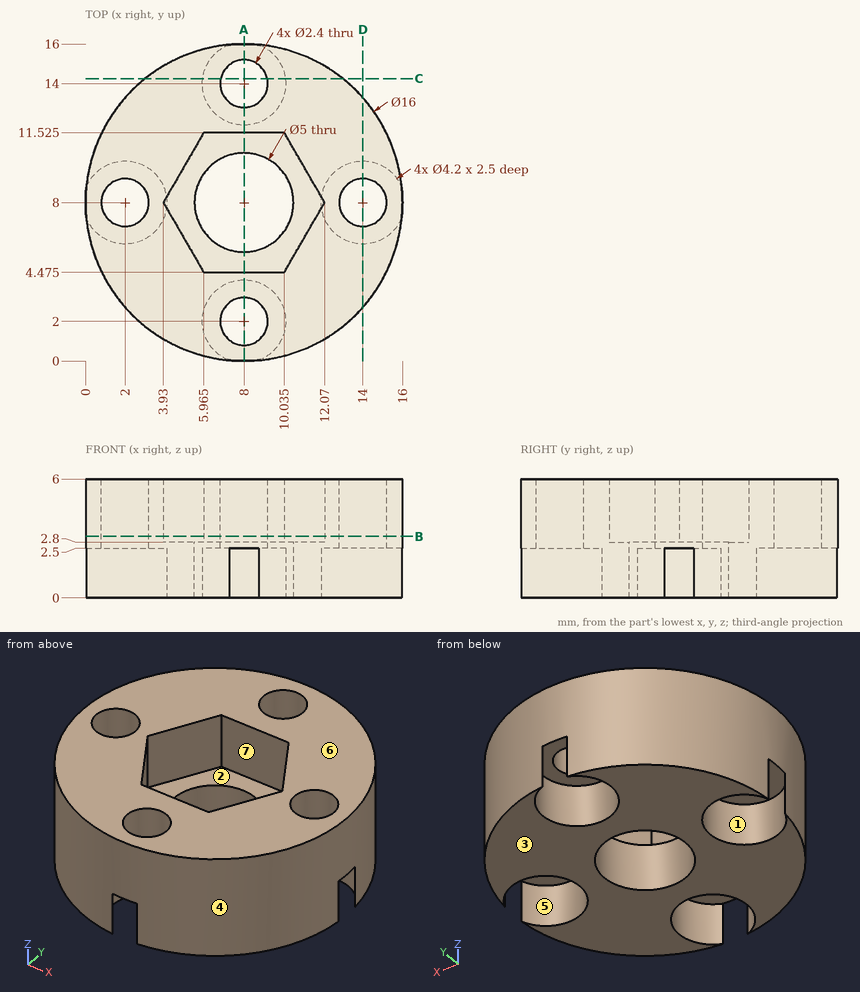
Design review of the part shown in the three views and the two pictorial views. Dimensions are in mm from the part's minimum x, y and z. A direction names the side the tool comes from. Round coordinates to 2 decimals unless told otherwise and drop trailing zeros. Order: outer loops, then holes, each group sorted by start corner. A loop starts at its lowest first (then second) coordinate and runs counter-clockwise, first axis right, second up. Notation, with made-up numbers: (61.5, 15.5) - (75.5, 15.5) arc R4 cw to (75.5, 20.5) - close; hole circle Ø8 at (33.5, 63.5). An arc over 180 degrees is marked (long way). Answer in a Markdown table with one row per item.
(1) Take a section at D-D on x = 14. Write out the cut boundary in (y, z), plus the area to 3 significant figures.
Result set:
| item | result |
|---|---|
| outline | (2.71, 0) - (5.9, 0) - (5.9, 2.5) - (6.8, 2.5) - (6.8, 6) - (2.71, 6) - close; (9.2, 2.5) - (10.1, 2.5) - (10.1, 0) - (13.29, 0) - (13.29, 6) - (9.2, 6) - close |
| area | 44.6 mm2 |
(2) Machinability: for the marked faces 5, 6 and 7, which of the approach directions +Z, -Z, +X, -X, +Y, -Y give a long, thin tool a straight path to every point of the face, cutting with its end or side? Answer none if there is none.
Result set:
| item | result |
|---|---|
| face 5 | -Z |
| face 6 | +Z, +X, -X, +Y, -Y |
| face 7 | +Z |
(3) Mouldability with a two-part tool opening along Y and no side actions: class the marked faces 1, 2, 3 and 4 as released by +Y, released by -Y, zero draft, split by the parting line, or undercut.
Result set:
| item | result |
|---|---|
| face 1 | undercut |
| face 2 | undercut |
| face 3 | zero draft |
| face 4 | split by the parting line |
(4) Clearance check with flat-ended pins moving along their axes: P1, Ø2, axis at x = 12, z = 1.5, coming from the +Y side; P2, Ø1.2, axis at x = 8, y = 1, coming from the -Z side; P3, Ø1, axis at y = 13, z = 2.5, coming from the +X side (1 decimal). State where each tip first meets the part, or that it passes through.
Result set:
| item | result |
|---|---|
| P1 | stops at y = 15.42 |
| P2 | stops at z = 2.5 |
| P3 | stops at x = 14.6 |
(5) Take a section at A-A on x = 8. Write out the cut boundary in (y, z) (1 decimal).
Result set:
| item | result |
|---|---|
| outline | (0, 2.5) - (0.8, 2.5) - (0.8, 6) - (0, 6) - close; (3.2, 2.5) - (4.1, 2.5) - (4.1, 0) - (5.5, 0) - (5.5, 2.8) - (4.5, 2.8) - (4.5, 6) - (3.2, 6) - close; (10.5, 0) - (11.9, 0) - (11.9, 2.5) - (12.8, 2.5) - (12.8, 6) - (11.5, 6) - (11.5, 2.8) - (10.5, 2.8) - close; (15.2, 2.5) - (16, 2.5) - (16, 6) - (15.2, 6) - close |
(6) Take a section at C-C on y = 14.25. Write out the cut boundary in (x, z) (1 decimal).
Result set:
| item | result |
|---|---|
| outline | (3, 0) - (5.9, 0) - (5.9, 2.5) - (6.8, 2.5) - (6.8, 6) - (3, 6) - close; (9.2, 2.5) - (10.1, 2.5) - (10.1, 0) - (13, 0) - (13, 6) - (9.2, 6) - close |
(7) For line 1 (Y direction, x = 8.5, z = 4) (1 decimal); line 2 (Z direction, x = 1.25, y = 9); line 3 (Z direction, x = 9.5, y = 5), list the stretches that pass through material, from the lowest coordinate up. Write a range as from..to.
Result set:
| item | result |
|---|---|
| line 1 | y = 0..0.9, 3.1..4.5, 11.5..12.9, 15.1..16 |
| line 2 | z = 2.5..6 |
| line 3 | z = 0..2.8 |
(8) Take a section at B-B on z = 3.1. Write out the cut boundary in (x, y) (1 decimal).
Result set:
| item | result |
|---|---|
| outline | circle Ø16 at (8, 8); hole circle Ø2.4 at (2, 8); hole (3.9, 8) - (6, 4.5) - (10, 4.5) - (12.1, 8) - (10, 11.5) - (6, 11.5) - close; hole circle Ø2.4 at (8, 2); hole circle Ø2.4 at (8, 14); hole circle Ø2.4 at (14, 8) |
